Build history of the part. All positions in model axes, mm. Face numbers are marked on the shaded views. Coordinates: 2 decimals unless noted, no trailing zeros. Loops run counter-clockwise (first coordinate to the right, second up) from the corner with the lowest first, then second, coordinate; pieces in that order, holes last. Notation, with made-up numbers: (-39, 36) - (-26, 36) arc R21 ccw to (-26, 48) - close; hole circle Ø2 at (70, -40). An arc over 180 degrees is marked (long way). One line per item, written item: value.
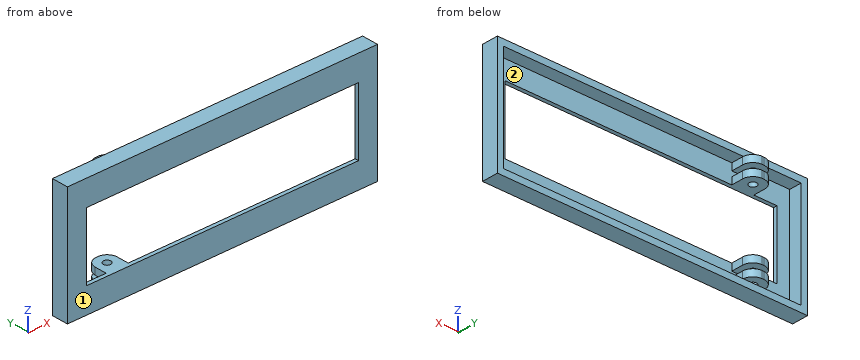
```python
from build123d import *

# Parameters (mm, degrees)
SKETCH4_W               = 2449.5
SKETCH4_H               = 930
SKETCH4_W_2             = 2149.5
SKETCH4_H_2             = 530
BOSS_EXTRUDE2_DEPTH     = 30
SKETCH6_W               = 2449.5
SKETCH6_H               = 930
SKETCH6_W_2             = 2349.5
SKETCH6_H_2             = 830
BOSS_EXTRUDE3_DEPTH     = 100
SKETCH8_W               = 174.417097876
SKETCH8_H               = 150
BOSS_EXTRUDE4_DEPTH     = 175
CUT_EXTRUDE1_DEPTH      = 680
CUT_EXTRUDE1_DEPTH_BACK = 150
SKETCH10_R              = 30
FILLET1_R               = 80
SKETCH12_W              = 40
SKETCH12_H              = 200
CUT_EXTRUDE2_DEPTH      = 184


with BuildPart() as part:
    # Sketch4 → Boss-Extrude2 (new body)
    with BuildSketch(Plane(origin=(0, 0, 0), x_dir=(1, 0, 0), z_dir=(0, 1, 0))):
        with Locations((2350.564429087, 865.22075714)):
            Rectangle(SKETCH4_W, SKETCH4_H)
        with Locations((2350.564429087, 865.22075714)):
            Rectangle(SKETCH4_W_2, SKETCH4_H_2, mode=Mode.SUBTRACT)
    extrude(amount=BOSS_EXTRUDE2_DEPTH)

    # Sketch6 → Boss-Extrude3 (add)
    with BuildSketch(Plane(origin=(0, 30, 0), x_dir=(1, 0, 0), z_dir=(0, 1, 0))):
        with Locations((2350.564429087, 865.22075714)):
            Rectangle(SKETCH6_W, SKETCH6_H)
        with Locations((2350.564429087, 865.22075714)):
            Rectangle(SKETCH6_W_2, SKETCH6_H_2, mode=Mode.SUBTRACT)
    extrude(amount=BOSS_EXTRUDE3_DEPTH)

    # Sketch8 → Boss-Extrude4 (add)
    with BuildSketch(Plane(origin=(0, 30, 0), x_dir=(1, 0, 0), z_dir=(0, 1, 0))):
        with Locations((1546.094821657, 1205.22075714)):
            Rectangle(SKETCH8_W, SKETCH8_H)
        with Locations((1546.094821657, 525.22075714)):
            Rectangle(SKETCH8_W, SKETCH8_H)
    extrude(amount=BOSS_EXTRUDE4_DEPTH)

    # Sketch10 → Cut-Extrude1 (cut, two sides: drawn at the far end of the back side and taken through both)
    with BuildSketch(Plane.XY.offset(-1130.22075714).offset(-CUT_EXTRUDE1_DEPTH_BACK)):
        with Locations(Location((1544.625999864, 116.419579706, 0), (0, 0, 180))):
            Circle(SKETCH10_R)
    extrude(amount=CUT_EXTRUDE1_DEPTH + CUT_EXTRUDE1_DEPTH_BACK, mode=Mode.SUBTRACT)

    # Fillet1
    # the kernel refuses this fillet: 80 mm, written as the material it takes off along each edge
    with BuildSketch(Plane(origin=(1633.303370595, 205, -1280.22075714), x_dir=(0, -1, 0), z_dir=(0, 0, 1)), Plane(origin=(1458.886272719, 205, -450.22075714), x_dir=(0, -1, 0), z_dir=(0, 0, -1))) as fillet1_piece_1:
        with BuildLine():
            CenterArc((FILLET1_R, -FILLET1_R), FILLET1_R, 90, 90)
            Line((0, -FILLET1_R), (0, 0))
            Line((0, 0), (FILLET1_R, 0))
        make_face()
    extrude(amount=350, mode=Mode.SUBTRACT)
    with BuildSketch(Plane(origin=(1458.886272719, 205, -930.22075714), x_dir=(1, 0, 0), z_dir=(0, 0, -1)), Plane(origin=(1633.303370595, 205, -800.22075714), x_dir=(-1, 0, 0), z_dir=(0, 0, 1))) as fillet1_piece_2:
        with BuildLine():
            CenterArc((FILLET1_R, FILLET1_R), FILLET1_R, 180, 90)
            Line((0, FILLET1_R), (0, 0))
            Line((0, 0), (FILLET1_R, 0))
        make_face()
    extrude(amount=350, mode=Mode.SUBTRACT)

    # Sketch12 → Cut-Extrude2 (cut)
    with BuildSketch(Plane(origin=(1633.303370595, 0, 0), x_dir=(0, 0, -1), z_dir=(1, 0, 0))):
        with Locations((1205.22075714, 130)):
            Rectangle(SKETCH12_W, SKETCH12_H)
        with Locations((525.22075714, 130)):
            Rectangle(SKETCH12_W, SKETCH12_H)
    extrude(amount=-CUT_EXTRUDE2_DEPTH, mode=Mode.SUBTRACT)


solid = part.part
```
Item 1: Cut at A-A, the plane y = 58. Write the cut outline in (x, z).
Check result:
outline: (1125.81, -1330.22) - (3575.31, -1330.22) - (3575.31, -400.22) - (1125.81, -400.22) - close; (1458.89, -1185.22) - (1633.3, -1185.22) - (1633.3, -1130.22) - (1458.89, -1130.22) - close; (1458.89, -600.22) - (1633.3, -600.22) - (1633.3, -545.22) - (1458.89, -545.22) - close; hole (1175.81, -1280.22) - (1458.89, -1280.22) - (1458.89, -1225.22) - (1633.3, -1225.22) - (1633.3, -1280.22) - (3525.31, -1280.22) - (3525.31, -450.22) - (1633.3, -450.22) - (1633.3, -505.22) - (1458.89, -505.22) - (1458.89, -450.22) - (1175.81, -450.22) - close
Item 2: Cut at D-D, the plane y = 168.5. Write the cut outline in (x, z).
Check result:
outline: (1471.75, -1280.22) - (1620.44, -1280.22) - (1620.44, -1225.22) - (1471.75, -1225.22) - close; (1471.75, -1185.22) - (1620.44, -1185.22) - (1620.44, -1130.22) - (1471.75, -1130.22) - close; (1471.75, -600.22) - (1620.44, -600.22) - (1620.44, -545.22) - (1471.75, -545.22) - close; (1471.75, -505.22) - (1620.44, -505.22) - (1620.44, -450.22) - (1471.75, -450.22) - close
Item 3: Pull direction X, two halves, no side cores. Call the marked faces 1 and 2: released by +X, released by -X, zero draft, split by the parting line, or undercut.
Check result:
face 1: zero draft
face 2: undercut
Item 4: Cut at C-C, the plane z = -879. Write the cut outline in (x, y), then the cut area to 3 significant figures.
Check result:
outline: (1125.81, 0) - (1275.81, 0) - (1275.81, 30) - (1175.81, 30) - (1175.81, 130) - (1125.81, 130) - close; (3425.31, 0) - (3575.31, 0) - (3575.31, 130) - (3525.31, 130) - (3525.31, 30) - (3425.31, 30) - close
area: 19,000 mm^2
Item 5: Probe probe 1 along X at (y, z) = (68, -453.5); probe 2 along X at (y, z) = (122.5, -510); probe 3 along Z at (x, y) = (3081, 70). List the from-to ranges inside material, lowest first. Write a range as from..to.
Check result:
probe 1: x = 1125.81..1175.81, 1458.89..1633.3, 3525.31..3575.31
probe 2: x = 1125.81..1175.81, 3525.31..3575.31
probe 3: z = -1330.22..-1280.22, -450.22..-400.22
Item 6: Cut at B-B, the plane x = 2324. Write the cut outline in (y, z).
Check result:
outline: (0, -1330.22) - (130, -1330.22) - (130, -1280.22) - (30, -1280.22) - (30, -1130.22) - (0, -1130.22) - close; (0, -600.22) - (30, -600.22) - (30, -450.22) - (130, -450.22) - (130, -400.22) - (0, -400.22) - close
